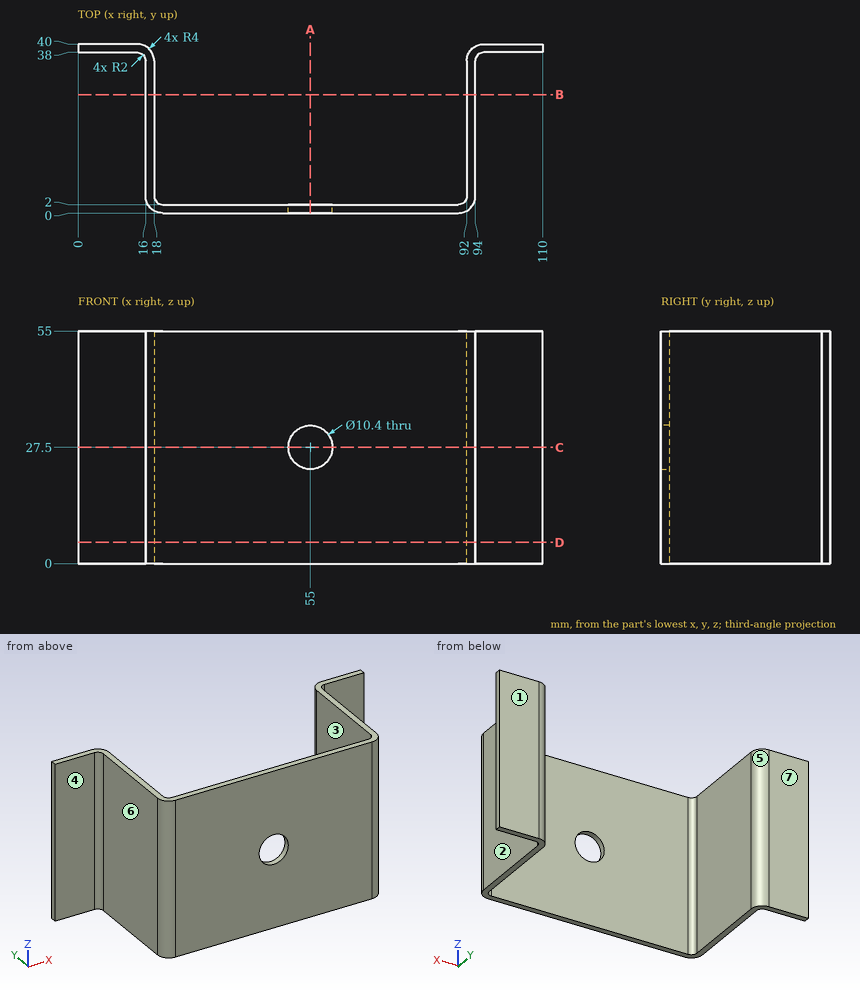
Part print with two shaded views. Sizes in mm from the minimum x, y, z corner. A direction names the side the tool comes from. Round coordinates to 2 decimals unless told otherwise and drop trailing zeros. Loops run counter-clockwise (first coordinate to the right, second up) from the corner with the lowest first, then second, coordinate; pieces in that order, holes last. Notation, with made-up numbers: (-23.5, -28) - (-2.5, -28) arc R21 ccw to (-2.5, -1) - close; hole circle Ø2 at (-23, 29.25). An arc over 180 degrees is marked (long way). Answer as a JSON object with one key per item and string values.
Item 1: Band-saw the part on B-B on y = 28. List the corners of the cut face in (x, z), plus the area to 3 significant figures.
Output:
{"outline": "(16, 0) - (18, 0) - (18, 55) - (16, 55) - close; (92, 0) - (94, 0) - (94, 55) - (92, 55) - close", "area": "220 mm2"}
Item 2: Pull direction X, two halves, no side cores. Call the marked faces 5, 6 and 7: pulls with the +X half, pulls with the -X half, needs draft (parallel to the pull), parting line crosses it, or undercut.
Output:
{"face 5": "undercut", "face 6": "pulls with the -X half", "face 7": "needs draft"}
Item 3: Band-saw the part on C-C on z = 27.5. List the corners of the cut face in (x, y).
Output:
{"outline": "(0, 38) - (14, 38) arc R2 cw to (16, 36) - (16, 4) arc R4 ccw to (20, 0) - (49.8, 0) - (49.8, 2) - (20, 2) arc R2 cw to (18, 4) - (18, 36) arc R4 ccw to (14, 40) - (0, 40) - close; (60.2, 0) - (90, 0) arc R4 ccw to (94, 4) - (94, 36) arc R2 cw to (96, 38) - (110, 38) - (110, 40) - (96, 40) arc R4 ccw to (92, 36) - (92, 4) arc R2 cw to (90, 2) - (60.2, 2) - close"}
Item 4: Tool access for the marked faces 1, 2, 3 and 4: list every direction of +Z, -Z, +X, -X, +Y, -Y with a clear straight run to the whole face (end or side of a thin tool).
Output:
{"face 1": "+Z, -Z, +X, -X, +Y", "face 2": "+Z, -Z, +X, -Y", "face 3": "+Z, -Z, +Y", "face 4": "+Z, -Z, -X, -Y"}
Item 5: Wall check: L1, parallel to X at y = 8, z = 50.5; L2, parallel to X at y = 0.55, z = 27.5; L3, parallel to Y at x = 61.5, z = 30.5. Give the ranges that are in metal, low to high.
Output:
{"L1": "16 to 18, 92 to 94", "L2": "17.98 to 49.8, 60.2 to 92.02", "L3": "0 to 2"}
Item 6: Band-saw the part on A-A on x = 55. List the corners of the cut face in (y, z).
Output:
{"outline": "(0, 0) - (2, 0) - (2, 22.3) - (0, 22.3) - close; (0, 32.7) - (2, 32.7) - (2, 55) - (0, 55) - close"}
Item 7: Band-saw the part on D-D on z = 5. List the corners of the cut face in (x, y), plus the area to 3 significant figures.
Output:
{"outline": "(0, 38) - (14, 38) arc R2 cw to (16, 36) - (16, 4) arc R4 ccw to (20, 0) - (90, 0) arc R4 ccw to (94, 4) - (94, 36) arc R2 cw to (96, 38) - (110, 38) - (110, 40) - (96, 40) arc R4 ccw to (92, 36) - (92, 4) arc R2 cw to (90, 2) - (20, 2) arc R2 cw to (18, 4) - (18, 36) arc R4 ccw to (14, 40) - (0, 40) - close", "area": "362 mm2"}
Item 8: Pin check, flat tips, straight feed: pin 1 (9.5 mm diameter, centred on y = 15, z = 23.5, fed in from -X); pin 2 (15.5 mm diameter, centred on x = 6, z = 39, fed in from -Y); pin 3 (4 mm diameter, centred on y = 6.5, z = 25, fed in from +X). Stop position of each tip, or through.
Output:
{"pin 1": "x = 16", "pin 2": "y = 38", "pin 3": "x = 94"}
